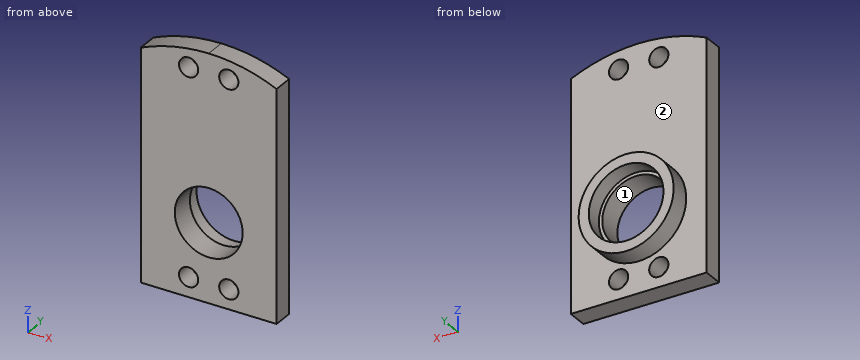
from build123d import *

# Parameters (mm, degrees)
SKETCH1_W             = 31.75
SKETCH1_H             = 57.15
BOSS_EXTRUDE1_DEPTH   = 4.7625
SKETCH2_R             = 11.1125
BOSS_EXTRUDE2_DEPTH   = 4.7625
SKETCH3_R             = 8.73125
CUT_EXTRUDE1_DEPTH    = 3.81
SKETCH4_R             = 7.9375
CUT_EXTRUDE2_DEPTH    = 7.9375
F_8_CLEARANCE_HOLE2_D = 4.4958
CUT_EXTRUDE3_DEPTH    = 5.7625


with BuildPart() as part:
    # Sketch1 → Boss-Extrude1 (new body)
    with BuildSketch(Plane(origin=(0, 0, 0), x_dir=(1, 0, 0), z_dir=(0, 1, 0))):
        Rectangle(SKETCH1_W, SKETCH1_H)
    extrude(amount=BOSS_EXTRUDE1_DEPTH)

    # Sketch2 → Boss-Extrude2 (add)
    with BuildSketch(Plane(origin=(0, 4.7625, 0), x_dir=(1, 0, 0), z_dir=(0, 1, 0))):
        with Locations((0, 10.15000002)):
            Circle(SKETCH2_R)
    extrude(amount=BOSS_EXTRUDE2_DEPTH)

    # Sketch3 → Cut-Extrude1 (cut)
    with BuildSketch(Plane(origin=(0, 9.525, 0), x_dir=(1, 0, 0), z_dir=(0, 1, 0))):
        with Locations((0, 10.15000002)):
            Circle(SKETCH3_R)
    extrude(amount=-CUT_EXTRUDE1_DEPTH, mode=Mode.SUBTRACT)

    # Sketch4 → Cut-Extrude2 (cut)
    with BuildSketch(Plane.XZ):
        with Locations((0, -10.15000002)):
            Circle(SKETCH4_R)
    extrude(amount=-CUT_EXTRUDE2_DEPTH, mode=Mode.SUBTRACT)

    # #8 Clearance Hole2 (through all)
    with Locations(Plane(origin=(0, 0, 0), x_dir=(-1, 0, 0), z_dir=(0, -1, 0))):
        with Locations((-4.7, 24.00000002), (4.7, -23.99999998), (4.7, 24.00000002), (-4.7, -23.99999998)):
            Hole(F_8_CLEARANCE_HOLE2_D / 2)

    # Sketch8 → Cut-Extrude3 (cut, through all)
    with BuildSketch(Plane(origin=(0, 4.7625, 0), x_dir=(1, 0, 0), z_dir=(0, 1, 0))):
        with BuildLine():
            ThreePointArc((15.875, -25.171523185), (8.117870402, -27.7145719), (0, -28.575))
            Line((0, -28.575), (15.875, -28.575))
            Line((15.875, -28.575), (15.875, -25.171523185))
        make_face()
        with BuildLine():
            ThreePointArc((0, -28.575), (-8.117870402, -27.7145719), (-15.875, -25.171523185))
            Line((-15.875, -25.171523185), (-15.875, -28.575))
            Line((-15.875, -28.575), (0, -28.575))
        make_face()
    extrude(amount=-CUT_EXTRUDE3_DEPTH, mode=Mode.SUBTRACT)


solid = part.part
Part model, mm, in its own coordinate system. Face numbers are marked on the shaded views. Coordinates: 2 decimals unless noted, no trailing zeros. Order: outer loops, then holes, each group sorted by start corner. A loop starts at its lowest first (then second) coordinate and runs counter-clockwise, first axis right, second up. Notation, with made-up numbers: M -26.75,-19.5 L 30.25,-19.5 A25 ccw 30.25,-4.5 Z; hole C -6.5,27.5 d9. An arc over 180 degrees is marked long. Use a Markdown table: item, result.
(1) Cut at A-A on y = 2.5. State how many separate pieces and enclosed holes the cut face has, then the cut area to 3 significant figures.
A:
| item | result |
|---|---|
| separate pieces | 1 |
| enclosed holes | 5 |
| area | 1,520 mm^2 |
(2) Cut at D-D on z = -10.15. Write the cut outline in (x, y) (1 decimal).
A:
| item | result |
|---|---|
| outline | M -15.9,0 L -7.9,0 L -7.9,5.7 L -8.7,5.7 L -8.7,9.5 L -11.1,9.5 L -11.1,4.8 L -15.9,4.8 Z; M 7.9,0 L 15.9,0 L 15.9,4.8 L 11.1,4.8 L 11.1,9.5 L 8.7,9.5 L 8.7,5.7 L 7.9,5.7 Z |
(3) Pull direction X, two halves, no side cores. Call the marked faces 1 and 2: released by +X, released by -X, zero draft, split by the parting line, or undercut.
A:
| item | result |
|---|---|
| face 1 | undercut |
| face 2 | zero draft |
(4) Cut at B-B on z = -24. Write the cut outline in (x, y) (1 decimal).
A:
| item | result |
|---|---|
| outline | M -15.9,0 L -6.9,0 L -6.9,4.8 L -15.9,4.8 Z; M -2.5,0 L 2.5,0 L 2.5,4.8 L -2.5,4.8 Z; M 6.9,0 L 15.9,0 L 15.9,4.8 L 6.9,4.8 Z |
(5) Flat gauge pins, fed straight in: pin 1 (3.5 mm diameter, centred on x = -4.7, z = -24, fed in from +Y); pin 2 (4 mm diameter, centred on x = -7.5, y = 8.5, fed in from +Z); pin 3 (7 mm diameter, centred on x = 4.7, z = 24, fed in from -Y); pin 4 (8 mm diameter, centred on x = -2, z = 20, fed in from +Y). Where does each tip first touch, or does it go through?
A:
| item | result |
|---|---|
| pin 1 | passes through |
| pin 2 | stops at z = -0.49 |
| pin 3 | stops at y = 0 |
| pin 4 | stops at y = 4.76 |
(6) Cut at C-C on x = -1.5. Write the cut outline in (y, z) (1 decimal), then the cut area to 3 significant figures.
A:
| item | result |
|---|---|
| outline | M 0,-28.6 L 4.8,-28.6 L 4.8,-21.2 L 9.5,-21.2 L 9.5,-18.8 L 5.7,-18.8 L 5.7,-17.9 L 0,-17.9 Z; M 0,-2.4 L 5.7,-2.4 L 5.7,-1.5 L 9.5,-1.5 L 9.5,0.9 L 4.8,0.9 L 4.8,28.5 L 0,28.5 Z |
| area | 222 mm^2 |
(7) Probe L1, parallel to X at y = 2.45, z = 24 (3 decimals); L2, parallel to X at y = 4, z = -10.15 (1 decimal); L3, parallel to Z at x = -4.7, y = 2.85 (3 decimals). List the from-to ranges inside material, lowest first.
A:
| item | result |
|---|---|
| L1 | x = -15.875 to -6.948, -2.452 to 2.452, 6.948 to 15.875 |
| L2 | x = -15.9 to -7.9, 7.9 to 15.9 |
| L3 | z = -28.575 to -26.248, -21.752 to -16.546, -3.754 to 21.752, 26.248 to 28.289 |
